Can you work these out from the model? Positions are in its coordinate system, mm. Face numbers are marked on the shaded views. A direction names the side the tool comes from. Give positions to 0.01 mm unless a question says otherwise; leave off trailing zeros. Loops run counter-clockwise (first coordinate to the right, second up) from the corner with the lowest first, then second, coordinate; pieces in that order, holes last.
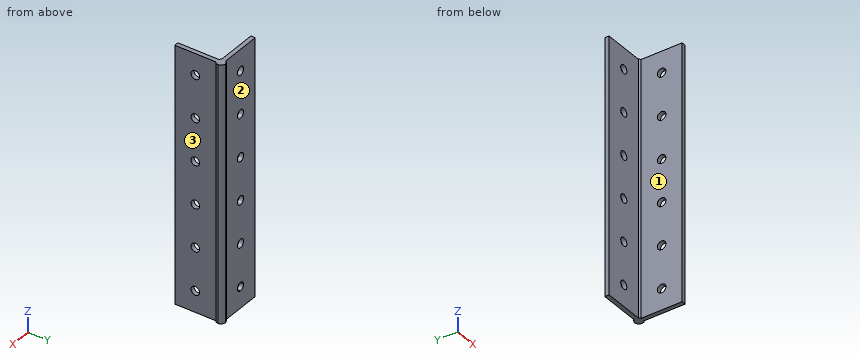
from build123d import *

# Parameters (mm, degrees)
F1_DEPTH = 76.2
F2_R     = 1.27
F3_DEPTH = 25.4
F4_R     = 1.27
F5_DEPTH = 25.4


with BuildPart() as f1:
    # F0 (on Top) → F1 (new body)
    with BuildSketch(Plane.XY):
        with BuildLine():
            ThreePointArc((0, 1.27), (0.0432742006, 1.5987001873), (0.1701477372, 1.905))
            Line((0.1701477372, 1.905), (-12.065, 1.905))
            Line((-12.065, 1.905), (-12.065, 0.635))
            Line((-12.065, 0.635), (0.1701477372, 0.635))
            ThreePointArc((0.1701477372, 0.635), (0.0432742006, 0.9412998127), (0, 1.27))
        make_face()
        with BuildLine():
            Line((1.905, -12.065), (1.905, 0.1701477372))
            ThreePointArc((1.905, 0.1701477372), (1.5987001873, 0.0432742006), (1.27, 0))
            ThreePointArc((1.27, 0), (0.9412998127, 0.0432742006), (0.635, 0.1701477372))
            Line((0.635, 0.1701477372), (0.635, -12.065))
            Line((0.635, -12.065), (1.905, -12.065))
        make_face()
        with BuildLine():
            ThreePointArc((1.905, 0.1701477372), (2.3698522628, 0.635), (2.54, 1.27))
            Line((2.54, 1.27), (1.905, 0.635))
            Line((1.905, 0.635), (1.905, 0.1701477372))
        make_face()
        with BuildLine():
            Line((1.27, 2.54), (2.54, 1.27))
            ThreePointArc((2.54, 1.27), (2.1680256121, 2.1680256121), (1.27, 2.54))
        make_face()
        Polygon((1.27, 1.27), (2.54, 1.27), (1.27, 2.54), align=None)
        Polygon((1.905, 0.635), (2.54, 1.27), (1.27, 1.27), (1.27, 0), align=None)
        with BuildLine():
            ThreePointArc((1.27, 0), (1.5987001873, 0.0432742006), (1.905, 0.1701477372))
            Line((1.905, 0.1701477372), (1.905, 0.635))
            Line((1.905, 0.635), (1.27, 0))
        make_face()
        with BuildLine():
            ThreePointArc((0.635, 0.1701477372), (0.9412998127, 0.0432742006), (1.27, 0))
            Line((1.27, 0), (0.635, 0.635))
            Line((0.635, 0.635), (0.635, 0.1701477372))
        make_face()
        with BuildLine():
            ThreePointArc((0.1701477372, 0.635), (0.3719743879, 0.3719743879), (0.635, 0.1701477372))
            Line((0.635, 0.1701477372), (0.635, 0.635))
            Line((0.635, 0.635), (0.1701477372, 0.635))
        make_face()
        with BuildLine():
            Line((0.635, 0.635), (0, 1.27))
            ThreePointArc((0, 1.27), (0.0432742006, 0.9412998127), (0.1701477372, 0.635))
            Line((0.1701477372, 0.635), (0.635, 0.635))
        make_face()
        Polygon((1.27, 0), (1.27, 1.27), (0, 1.27), (0.635, 0.635), align=None)
        Polygon((1.27, 1.27), (1.27, 2.54), (0.635, 1.905), (0, 1.27), align=None)
        with BuildLine():
            Line((0.635, 1.905), (0.1701477372, 1.905))
            ThreePointArc((0.1701477372, 1.905), (0.0432742006, 1.5987001873), (0, 1.27))
            Line((0, 1.27), (0.635, 1.905))
        make_face()
        with BuildLine():
            Line((0.635, 1.905), (1.27, 2.54))
            ThreePointArc((1.27, 2.54), (0.635, 2.3698522628), (0.1701477372, 1.905))
            Line((0.1701477372, 1.905), (0.635, 1.905))
        make_face()
    extrude(amount=F1_DEPTH)

    # F2 (on face) → F3 (cut)
    with BuildSketch(Plane.YZ.offset(1.905)):
        with Locations((-5.9474261314, 69.85)):
            Circle(F2_R)
        with Locations((-5.9474261314, 57.15)):
            Circle(F2_R)
        with Locations((-5.9474261314, 44.45)):
            Circle(F2_R)
        with Locations((-5.9474261314, 31.75)):
            Circle(F2_R)
        with Locations((-5.9474261314, 19.05)):
            Circle(F2_R)
        with Locations((-5.9474261314, 6.35)):
            Circle(F2_R)
    extrude(amount=-F3_DEPTH, mode=Mode.SUBTRACT)

    # F4 (on face) → F5 (cut)
    with BuildSketch(Plane(origin=(0, 1.905, 0), x_dir=(-1, 0, 0), z_dir=(0, 1, 0))):
        with Locations((5.9474261314, 69.85)):
            Circle(F4_R)
        with Locations((5.9474261314, 57.15)):
            Circle(F4_R)
        with Locations((5.9474261314, 44.45)):
            Circle(F4_R)
        with Locations((5.9474261314, 31.75)):
            Circle(F4_R)
        with Locations((5.9474261314, 19.05)):
            Circle(F4_R)
        with BuildLine():
            ThreePointArc((7.2174261314, 6.35), (5.0494005193, 7.2480256121), (5.9474261314, 5.08))
            ThreePointArc((5.9474261314, 5.08), (6.8454517435, 5.4519743879), (7.2174261314, 6.35))
        make_face()
    extrude(amount=-F5_DEPTH, mode=Mode.SUBTRACT)


solid = f1.part
(1) Will these pins go through, and if not, where does the flat tip stop? P1, Ø4, axis at x = -4, z = 19, coming from the -Y side (3 decimals); P2, Ø6, axis at y = -5, z = 44.5, coming from the -X side (3 decimals); P3, Ø3.5, axis at x = -5.95, z = 69.85, coming from the +Y side (3 decimals).
Returned:
P1: stops at y = 0.635
P2: stops at x = 0.635
P3: stops at y = 1.905
(2) Suppose I cut it at A-A on z = 44.45. List the corners of the cut face in (x, y) for me (3 decimals), plus the area to 3 significant figures.
Returned:
outline: (-12.065, 0.635) - (-7.217, 0.635) - (-7.217, 1.905) - (-12.065, 1.905) - close; (-4.677, 0.635) - (0.17, 0.635) arc R1.27 ccw to (0.635, 0.17) - (0.635, -4.677) - (1.905, -4.677) - (1.905, 0.17) arc R1.27 ccw (long way) to (0.17, 1.905) - (-4.677, 1.905) - close; (0.635, -12.065) - (1.905, -12.065) - (1.905, -7.217) - (0.635, -7.217) - close
area: 29.4 mm2
(3) Suppose I cut it at B-B on x = -1.75. List the corners of the cut face in (y, z) for me (3 decimals), plus the area to 3 significant figures.
Returned:
outline: (0.635, 0) - (1.905, 0) - (1.905, 76.2) - (0.635, 76.2) - close
area: 96.8 mm2
(4) Please list where these lines run through material, in increasing order: probe 1 along Y at (x, z) = (-11, 67) (3 decimals); probe 2 along X at (y, z) = (1.1, 69.85) (3 decimals).
Returned:
probe 1: y = 0.635 to 1.905
probe 2: x = -12.065 to -7.217, -4.677 to 2.529
(5) Which directions (+Z, -Z, +X, -X, +Y, -Y) give clear straight access to the entire face, cutting with the end or side of a thin tool? Please do the marked faces 1, 2 and 3.
Returned:
face 1: +Z, -Z, -X, -Y
face 2: +Z, -Z, -X, +Y
face 3: +Z, -Z, +X, -Y
